Autodesk Inventor part; units mm, degrees
ref_plane "YZ Plane" through (0, 0, 0) normal (1, 0, 0) x (0, 1, 0)
ref_plane "XZ Plane" through (0, 0, 0) normal (0, 1, 0) x (-1, 0, 0)
ref_plane "XY Plane" through (0, 0, 0) normal (0, 0, 1) x (1, 0, 0)
sketch "스케치1" plane through (0, 0, 0) normal (0, 1, 0) x (-1, 0, 0)
  line L0 (0, 0) -> (29.6, 0)
  line L1 (29.6, 0) -> (29.6, -55)
  line L2 (29.6, -55) -> (0, -55)
  line L3 (0, -55) -> (0, 0)
  dimension "d0" = 29.6
  dimension "d1" = 55
extrude "돌출1" add sketch "스케치1" along normal blind 3
sketch "스케치2" plane through (0, 3, 0) normal (0, 1, 0) x (1, 0, 0)
  line L0 (0, 55) -> (-29.6, 55)
  line L1 (-29.6, 55) -> (-29.6, 0)
  line L2 (-29.6, 0) -> (0, 0)
  line L3 (0, 0) -> (0, 55)
  line L4 (5.2, 0) -> (-34.8, 0)
  line L5 (-34.8, 0) -> (-34.8, 55)
  line L6 (-34.8, 55) -> (5.2, 55)
  line L7 (5.2, 55) -> (5.2, 0)
  line L8 (0, 55) -> (-29.6, 55)
  point P0 (-14.8, 0)
  point P1 (0, 55)
  point P2 (-29.6, 55)
  dimension "d4" = 40
  dimension "d5" = 20
extrude "돌출2" add sketch "스케치2" along normal blind 3
sketch "스케치3" plane through (5.2, 3, 0) normal (1, 0, 0) x (0, 0, -1)
  line L0 (0, 0) -> (55, 0)
  line L1 (55, 0) -> (55, 3)
  line L2 (0, 3) -> (55, 3)
  line L3 (0, 0) -> (0, 3)
  circle A0 centre (27.3, -7.4568) radius 9.5
  point P0 (0, -3)
  point P1 (33.1861, 0)
  point P2 (21.4139, 0)
  dimension "d8" = 19
extrude "돌출3" cut sketch "스케치3" against normal blind 3 contours A0 L0 picked at (27.9995, 0.6028)
fillet "모깎기1" radius 2 1 edges at (5.2, 5.0432, -27.3)
properties part number "motor cover1"
Input: part model. Units: mm. Frame: model coordinates. A direction names the side the tool comes from. Give positions to 0.01 mm unless a question says otherwise; leave off trailing zeros. Write each loop counter-clockwise with the first axis right and the second up, starting at its lowest first coordinate (ties: lowest second). Pieces come first, ordered by that corner, then holes. Notation, with made-up numbers: M -9.75,2.25 L 24.25,2.25 A23 ccw 24.25,19.25 Z; hole C 59.25,15.25 d7. An arc over 180 degrees is marked long. Use one line per item in the form item = value.
1. Reachability of faces 1 (the face through (2, 3, -28)), 2 (the face through (-29.6, 1, -27)), 3 (the face through (5.2, 4, -44)) from +Z, -Z, +X, -X, +Y, -Y: full face, straight path, thin tool, end or side. Return the list, or none.
Outcome:
face_1 = +Z, -Z, +X, -Y
face_2 = +Z, -Z, -X, -Y
face_3 = +Z, -Z, +X, +Y, -Y
2. Cut plane A-A on z = -4.5. Return loops of the section in (x, y), and give its area (3 significant figures).
Outcome:
outline = M -34.8,3 L -29.6,3 L -29.6,0 L 0,0 L 0,3 L 5.2,3 L 5.2,6 L -34.8,6 Z
area = 209 mm²
3. First-contact query: P1, Ø1.5, axis at y = 2, z = -33, coming from the -X side; P2, Ø2.5, axis at y = 1, z = -27, coming from the +X side; P3, Ø5.5, axis at x = -33, z = -26.5, coming from the -Y side. Flat tips, straight axial feed; report the tip coordinate or a pass-through.
Outcome:
P1 = -29.6
P2 = 0
P3 = 3
4. Cut plane B-B on y = 1.25. Return loops of the section in (x, z).
Outcome:
outline = M -29.6,-55 L 0,-55 L 0,0 L -29.6,0 Z
5. Ray query, L1, parallel to X at y = 0.75, z = -5; L2, parallel to Y at x = -32, z = -36.5; L3, parallel to Y at x = 3, z = -27.5. Return the intervals inside material, ascending.
Outcome:
L1 = -29.6 to 0
L2 = 3 to 6
L3 = 5.04 to 6
6. Mould query, pull axis Z, two halves, no side actions, for faces 4 (the face through (2.2, 4, -27)), 5 (the face through (-15, 3, 0)), 6 (the face through (-34.8, 4, -27)), 7 (the face through (2.707, 5.043, -27.389)). Classes: released by +Z, released by -Z, zero draft, split by the parting line, or undercut.
Outcome:
face_4 = undercut
face_5 = released by +Z
face_6 = zero draft
face_7 = undercut
